from build123d import *

# Parameters (mm, degrees)
OBR_T1_ANGLE                = 180.0000000000004
WYTNIJ_WYCI_GNI_CIE6_DEPTH  = 172.4642819948225
WYTNIJ_WYCI_GNI_CIE7_DEPTH  = 166.27116841238856
DODANIE_WYCI_GNI_CIE2_DEPTH = 100
WYTNIJ_WYCI_GNI_CIE8_DEPTH  = 172.45844977719824
WYCI_CIE_OBR_T2_ANGLE       = 90.0000000000002
WYTNIJ_WYCI_GNI_CIE9_DEPTH  = 172.45844977719824
SKORUPA2_T                  = -2


with BuildPart() as part:
    # Szkic1 → Obrót1 (revolve)
    with BuildSketch(Plane(origin=(0, 0, 0), x_dir=(0, 0, -1), z_dir=(1, 0, 0))):
        with BuildLine():
            Line((0, -55), (0, 55))
            Line((0, 55), (-75, 54.99999999999999))
            ThreePointArc((-75, 54.99999999999999), (-93.00537618869137, 1.139e-14), (-75, -54.99999999999999))
            Line((-75, -54.99999999999999), (0, -55))
        make_face()
    revolve(axis=Axis((0, -55, 0), (0, 1, 0)), revolution_arc=OBR_T1_ANGLE)

    # Szkic2 → Wytnij-wyciągnięcie6 (cut, through all)
    with BuildSketch(Plane.XZ.offset(54.99999999999998)):
        with BuildLine():
            Line((-50.14037658161271, 0), (-26.065901524307794, 0))
            Line((-26.065901524307794, 0), (-26.065901524307794, 75.00000000000003))
            Line((-26.065901524307794, 75.00000000000003), (0, 75.00000000000003))
            ThreePointArc((-7.11e-15, 75.00000000000004), (6.164498496803606, 74.74623039513706), (12.28728066433489, 73.98663888754419))
            ThreePointArc((12.287280664334872, 73.9866388875442), (66.51313822370639, 34.6554821584426), (67.6776695296636, -32.32233047033656))
            Line((67.6776695296636, -32.32233047033656), (87.35369951614506, -51.99836045681815))
            Line((87.35369951614506, -51.99836045681814), (99.7170587397922, -51.99836045681808))
            Line((99.7170587397922, -51.99836045681808), (99.7170587397922, 112.3930651923552))
            Line((99.71705873979221, 112.3930651923552), (-50.14037658161271, 112.3930651923552))
            Line((-50.14037658161271, 112.3930651923552), (-50.14037658161271, 0))
        make_face()
    extrude(amount=-WYTNIJ_WYCI_GNI_CIE6_DEPTH, mode=Mode.SUBTRACT)

    # Szkic6 → Wytnij-wyciągnięcie7 (cut, through all)
    with BuildSketch(Plane.XZ.offset(54.99999999999998)):
        with BuildLine():
            ThreePointArc((67.67766952966359, -32.32233047033659), (63.4396358173472, 40.00515725956293), (5.5067e-13, 75.00000000000003))
            Line((5.375e-13, 75.00000000000003), (-4.59e-15, 0))
            Line((0, 0), (17.677669529663717, 17.67766952966366))
            Line((17.677669529663717, 17.67766952966366), (67.6776695296636, -32.32233047033657))
        make_face()
    extrude(amount=-WYTNIJ_WYCI_GNI_CIE7_DEPTH, mode=Mode.SUBTRACT)

    # Szkic7 → Dodanie-wyciągnięcie2 (add)
    with BuildSketch(Plane(origin=(100, 0, 0), x_dir=(0, 0, -1), z_dir=(1, 0, 0))):
        Polygon((-60, -15.653786999192038), (-60, 14.34621300080796), (45.666627766936244, 29.346213000808905), (45.666627766936244, -30.653786999192953), align=None)
    extrude(amount=-DODANIE_WYCI_GNI_CIE2_DEPTH)

    # Szkic8 → Wycięcie-obrót1 (revolve, cut)
    with BuildSketch(Plane(origin=(0, 0, 0), x_dir=(0, 0, -1), z_dir=(1, 0, 0))):
        with BuildLine():
            Line((-74.9933330370107, 55.00000000000001), (-155.56349186104046, 55.00000000000001))
            ThreePointArc((-155.56349186104046, 55.00000000000001), (-165, 2.021e-14), (-155.56349186104046, -54.999999999999964))
            Line((-155.56349186104046, -54.999999999999964), (-74.99333303701071, -54.99999999999997))
            ThreePointArc((-74.99333303701071, -54.99999999999997), (-93, 1.139e-14), (-74.9933330370107, 55.00000000000001))
        make_face()
    revolve(axis=Axis((0, 0, 0), (0, 1, 0)), mode=Mode.SUBTRACT)

    # Szkic9 → Wytnij-wyciągnięcie8 (cut, through all)
    with BuildSketch(Plane.XZ.offset(54.99999999999998)):
        Polygon((-4.3e-16, -4.3e-16), (84.28181453760202, 84.28181453760173), (-46.691543450070924, 84.28181453760173), (-46.691543450070924, 0), align=None)
    extrude(amount=-WYTNIJ_WYCI_GNI_CIE8_DEPTH, mode=Mode.SUBTRACT)

    # Szkic10 → Wycięcie-obrót2 (revolve, cut)
    with BuildSketch(Plane(origin=(0, 0, 0), x_dir=(0, 0, -1), z_dir=(1, 0, 0))):
        with BuildLine():
            Line((-71.86967371569179, 55.00000000000001), (-106.6536450385077, 55.00000000000001))
            ThreePointArc((-106.6536450385077, 55.00000000000001), (-120, 1.47e-14), (-106.65364503850772, -54.99999999999998))
            Line((-106.65364503850772, -54.99999999999998), (-71.8696737156918, -54.99999999999998))
            ThreePointArc((-71.8696737156918, -54.99999999999998), (-90.5, 1.108e-14), (-71.86967371569179, 55.00000000000001))
        make_face()
    revolve(axis=Axis((0, 0, 0), (0, 1, 0)), revolution_arc=WYCI_CIE_OBR_T2_ANGLE, mode=Mode.SUBTRACT)

    # Szkic11 → Wytnij-wyciągnięcie9 (cut, through all)
    with BuildSketch(Plane.XZ.offset(54.99999999999998)):
        with BuildLine():
            ThreePointArc((25.000000000000004, -28), (17.67766952966355, -10.32233047033617), (-3.9815e-13, -2.9999999999999964))
            Line((0, -2.9999999999999964), (0, -28))
            Line((-1.9552e-13, -28), (-3.701e-13, -53))
            ThreePointArc((-6.7073e-13, -53), (17.67766952966345, -45.67766952966393), (25.000000000000004, -28.000000000000007))
        make_face()
        with BuildLine():
            Line((0, -28), (0, -2.9999999999999964))
            ThreePointArc((-3.9815e-13, -2.9999999999999964), (-25.000000000000004, -27.999999999999865), (-6.7073e-13, -53))
            Line((-3.701e-13, -53), (-1.9552e-13, -28))
        make_face()
    extrude(amount=-WYTNIJ_WYCI_GNI_CIE9_DEPTH, mode=Mode.SUBTRACT)

    # Skorupa2
    skorupa2_openings = [part.faces().sort_by_distance(p)[0] for p in [
        (63.613171512, -0.551610376, 60),
        (25, 0, -28),
        (21.502764512, -0.287252782, 21.502764512),
        (60.525104479, -22.455388981, 12.086510343),
        (60.727668941, 21.157570461, 12.017788444),
        (44.39246987, 39.229169277, -9.037130811),
        (0, 0, -1.5),
        (44.239594619, -39.899256445, -8.88425556),
    ]]
    offset(amount=SKORUPA2_T, openings=skorupa2_openings, kind=Kind.INTERSECTION)


solid = part.part
Model file for the job. Use its own axes, mm. A direction names the side the tool comes from. Give positions to 0.01 mm unless a question says otherwise; leave off trailing zeros. Loops run counter-clockwise (first coordinate to the right, second up) from the corner with the lowest first, then second, coordinate; pieces in that order, holes last.
1) Flat gauge pins, fed straight in: pin 1 Ø2 at (x, y) = (23.5, -4.5) entering from -Z; pin 2 Ø19 at (y, z) = (-21.5, -66) entering from +X; pin 3 Ø8 at (y, z) = (13, -41.5) entering from +X. Where does each tip first touch, or does it go through?
2) Saw through at D-D (x = 59). Write the cut outline in (y, z), plus the area to 3 significant figures.
3) Wall check: line 1 (Y direction, x = 49.5, z = -14.5); line 2 (X direction, y = 47.5, z = -60); line 3 (Z direction, x = 65, y = -9). Give the ranges that are in metal, low to high.
4) Pull direction Y, two halves, no side cores. Call faces 5 (the flat face through (85.42, -22.39, 12.55)), 6 (the flat face through (51.782, -53.665, -16.427)), 7 (the flat face through (34, -53, -29)): +Y half, -Y half, draft (parallel to the pull), parting line (faces both ways), or undercut.
5) Saw through at A-A (x = 12). Write the cut outline in (y, z).
6) Saw through at B-B (z = -28). Write the cut outline in (x, y), plus the area to 3 significant figures.
7) Saw through at C-C (y = -7). Write the cut outline in (x, z).
8) Tool access for faces 1 (the flat face through (91, 0, 0)), 2 (the flat face through (2, 1, -68)), 3 (the flat face through (0, 1, -69)), 4 (the flat face through (89, 0, -2)): list every direction of +Z, -Z, +X, -X, +Y, -Y with a clear straight run to the whole face (end or side of a thin tool).
Answer block:
1. pin 1: stops at z = -90.13
1. pin 2: stops at x = 71.13
1. pin 3: stops at x = 84.2
2. outline: (-55, -46.29) arc R71.89 ccw to (55, -46.29) - (55, -23.64) - (53, -23.64) - (53, -44.62) arc R69.28 cw to (-53, -44.62) - (-53, -23.64) - (-55, -23.64) - close
2. area: 408 mm2
3. line 1: y = -55 to -53, 53 to 55
3. line 2: x = 0 to 2, 49.24 to 52.85
3. line 3: z = -65.9 to -63.05, 59.38 to 60
4. face 5: -Y half
4. face 6: draft
4. face 7: undercut
5. outline: (-55, -74.03) arc R92.22 ccw to (55, -74.03) - (55, -49.93) - (53, -49.93) - (53, -72.99) arc R90.21 cw to (-53, -72.99) - (-53, -49.93) - (-55, -49.93) - close; (-55, -6.07) - (-53, -6.07) - (-53, 12) - (-55, 12) - close; (53, -6.07) - (55, -6.07) - (55, 12) - (53, 12) - close
6. outline: (25, -55) - (63.36, -55) - (63.36, -53) - (25, -53) - close; (25, 53) - (63.36, 53) - (63.36, 55) - (25, 55) - close; (81.88, -28.15) - (84.1, -28.15) arc R88.68 ccw to (84.53, 26.84) - (82.32, 26.84) arc R86.59 cw to start
6. area: 271 mm2
7. outline: (0, -92.74) arc R92.74 ccw to (92.74, 0) - (90.23, 0) arc R90.23 ccw to (67.39, 60) - (64.68, 60) arc R88.22 cw to (88.2, -2) - (90.71, -2) arc R90.73 cw to (2, -90.71) - (2, -52.92) arc R25 cw to (0, -53) - close
8. face 1: +Z, +X
8. face 2: +Z
8. face 3: +Z, -Z, -X, +Y, -Y
8. face 4: -X
